Can you work these out from the model? Positions are in its coordinate system, mm. A direction names the side the tool comes from. Give positions to 0.01 mm unless a question says otherwise; leave off trailing zeros. Loops run counter-clockwise (first coordinate to the right, second up) from the corner with the lowest first, then second, coordinate; pieces in that order, holes last. Notation, with made-up numbers: (62.5, 36) - (81.5, 36) arc R20 ccw to (81.5, 51) - close; hole circle Ø2 at (-11.75, 25.5). An arc over 180 degrees is marked (long way). Answer as a JSON object with one key per item and string values. Group by question number.
Item 1: Thinking about a two-plate mould opening in X: for faces 4 (the cylindrical face through (0.964, -2.841, 0.154)), 5 (the flat face through (-3, 2, -7)), 6 (the cylindrical face through (-5.689, -1.908, -7.451)), 7 (the flat face through (-1, -3, -11)), which applies, pulls with the +X half, pulls with the -X half, needs draft (parallel to the pull), parting line crosses it, or undercut?
Item 2: Will these pins go through, and if not, where does the flat tip stop? pin 1 (1.5 mm diameter, centred on x = 0.5, z = -3.5, fed in from +Y); pin 2 (2.5 mm diameter, centred on y = 1.5, z = 8.5, fed in from +X); pin 3 (3.5 mm diameter, centred on y = 1.5, z = -6.5, fed in from +X).
Item 3: Which directions (+Z, -Z, +X, -X, +Y, -Y) give clear straight access to the entire face, cutting with the end or side of a thin tool? Please do faces 1 (the flat face through (5, 0, 0)), 2 (the flat face through (-3, -2, 4)), 3 (the cylindrical face through (-4, 4, -7)).
Item 4: Suppose I cut it at D-D on y = -6.25. Write out the boundary of the cut face in (x, z), and give its area (3 significant figures).
Item 5: Suppose I cut it at C-C on x = 3.75. Write out the boundary of the cut face in (y, z).
Item 6: Please list where these lines run through material, in increasing order: L1, parallel to Z at x = -1.25, y = -5.75; L2, parallel to X at y = -0.5, z = -5.25; L3, parallel to X at y = -5, z = 0.5.
Item 7: Suppose I cut it at B-B on z = -6.75. Write out the boundary of the cut face in (x, y).
Item 8: Suppose I cut it at A-A on y = -2.5. Write out the boundary of the cut face in (x, z).
from build123d import *

# Parameters (mm, degrees)
PAD_DEPTH    = 11
POCKET_DEPTH = 4
FILLET_R     = 1
FILLET001_R  = 2


with BuildPart() as part:
    # Sketch → Pad (new body, symmetric)
    with BuildSketch(Plane.XY):
        with BuildLine():
            ThreePointArc((-3, 0), (0, -3), (3, 0))
            Line((3, 0), (8, 0))
            Line((8, 0), (0, -8))
            Line((0, -8), (0, -6))
            ThreePointArc((-3, 5.196152), (-5.795555, -1.552914), (0, -6))
            Line((-3, 5.196152), (-3, 0))
        make_face()
    extrude(amount=PAD_DEPTH, both=True)

    # Sketch001 → Pocket (cut, symmetric)
    with BuildSketch(Plane.XY):
        with BuildLine():
            ThreePointArc((0.45045, 7.486461), (-7.496614, 0.225327), (0, -7.5))
            Line((0, -2.5), (0, -7.5))
            ThreePointArc((0.45045, 2.459084), (-2.48975, 0.226152), (0, -2.5))
            Line((0.45045, 2.459084), (0.45045, 7.486461))
        make_face()
    extrude(amount=POCKET_DEPTH, both=True, mode=Mode.SUBTRACT)

    # Fillet
    fillet_edges = [part.edges().sort_by_distance(p)[0] for p in [
        (-3, 5.196152, 7.5),
        (-3, 5.196152, -7.5),
    ]]
    fillet(fillet_edges, radius=FILLET_R)

    # Fillet001
    fillet001_edges = [part.edges().sort_by_distance(p)[0] for p in [
        (0, -6, -7.5),
        (0, -6, 7.5),
    ]]
    fillet(fillet001_edges, radius=FILLET001_R)


solid = part.part
Worked out:
{
 "1": {"face 4": "undercut", "face 5": "pulls with the +X half", "face 6": "pulls with the -X half", "face 7": "needs draft"},
 "2": {"pin 1": "stops at y = -2.73", "pin 2": "stops at x = -3", "pin 3": "stops at x = 8"},
 "3": {"face 1": "+Z, -Z, +X, +Y", "face 2": "-X, +Y, -Y", "face 3": "+Z, -Z, +Y"},
 "4": {"outline": "(-0.67, -11) - (1.75, -11) - (1.75, 11) - (-0.67, 11) - (-0.67, 4) - (0, 4) - (0, -4) - (-0.67, -4) - close", "area": "47.9 mm2"},
 "5": {"outline": "(-4.25, -11) - (0, -11) - (0, 11) - (-4.25, 11) - close"},
 "6": {"L1": "z = -11 to -4, 4 to 11", "L2": "x = -5.98 to -2.96, 2.96 to 7.5", "L3": "x = 0 to 3"},
 "7": {"outline": "(-4.8, 3.6) arc R6 ccw to (-1.5, -5.81) arc R2 cw to (0, -7.75) - (0, -8) - (8, 0) - (3, 0) arc R3 cw to (-3, 0) - (-3, 3) arc R1 ccw to start"},
 "8": {"outline": "(-5.45, -11) - (-1.66, -11) - (-1.66, -4) - (-5.45, -4) - close; (-5.45, 4) - (-1.66, 4) - (-1.66, 11) - (-5.45, 11) - close; (1.66, -11) - (5.5, -11) - (5.5, 11) - (1.66, 11) - close"}
}
